Autodesk Inventor part; units mm, degrees
ref_plane "YZ Plane" through (0, 0, 0) normal (1, 0, 0) x (0, 1, 0)
ref_plane "XZ Plane" through (0, 0, 0) normal (0, 1, 0) x (-1, 0, 0)
ref_plane "XY Plane" through (0, 0, 0) normal (0, 0, 1) x (1, 0, 0)
sketch "Sketch1" plane through (0, 0, 0) normal (0, 0, 1) x (1, 0, 0)
  circle A0 centre (0, 0) radius 19.05
  circle A1 centre (0, 0) radius 9.906
  circle A2 centre (0, 0) radius 3
  dimension "d0" = 38.1
  dimension "d1" = 19.812
  dimension "d2" = 6
extrude "Extrusion1" add sketch "Sketch1" along normal blind 34.417 contours A0 | A1 | A2
extrude "Extrusion2" add sketch "Sketch1" against normal blind 5.207 contours A1
extrude "Extrusion3" add sketch "Sketch1" against normal blind 17.5768 contours A2
fillet "Fillet1" radius 1.5875 1 edges at (-19.05, 0, 34.417)
properties part number "OpticalRotaryEncoder"
Could you check a few things on this model? Use its own coordinates, in mm. A direction names the side the tool comes from. Give positions to 0.01 mm unless a question says otherwise; leave off trailing zeros. Order: outer loops, then holes, each group sorted by start corner. A loop starts at its lowest first (then second) coordinate and runs counter-clockwise, first axis right, second up. Notation, with made-up numbers: (79.25, 66.5) - (111.25, 66.5) arc R28 ccw to (111.25, 104.5) - close; hole circle Ø2 at (47, -6). An arc over 180 degrees is marked (long way). Return JSON: item names as keys, results as strings. Group by question number.
Q1. Which directions (+Z, -Z, +X, -X, +Y, -Y) give clear straight access to the entire face, cutting with the end or side of a thin tool? Please do faces 1 (the face through (-1.29, 9.82, -2.57)), 2 (the face through (0, 0, 34.417)).
Q2. Suppose I cut it at D-D, the plane z = -13. Please give me the cut outline in (x, y), and give its area (3 significant figures).
Q3. Suppose I cut it at C-C, the plane z = -2. Please give me the cut outline in (x, y).
Q4. Will these pins go through, and if not, where does the flat tip stop? pin 1 Ø3 at (x, z) = (-8, 16) entering from -Y; pin 2 Ø12 at (x, y) = (12.5, -14) entering from -Z; pin 3 Ø4 at (y, z) = (-0.5, -4.5) entering from -X.
Q5. Please list where these lines run through material, in increasing order: line 1 along Z through (x, y) = (-2.5, 12.5); line 2 along Z through (x, y) = (-0.5, 4); line 3 along Y through (x, z) = (0, -3). Write a range as [from, to].
Resolved:
{
 "1": {"face 1": "-Z", "face 2": "+Z, +X, -X, +Y, -Y"},
 "2": {"outline": "circle Ø6 at (0, 0)", "area": "28.3 mm2"},
 "3": {"outline": "circle Ø19.81 at (0, 0)"},
 "4": {"pin 1": "stops at y = -17.91", "pin 2": "stops at z = 0", "pin 3": "stops at x = -9.91"},
 "5": {"line 1": "z = [0, 34.42]", "line 2": "z = [-5.21, 34.42]", "line 3": "y = [-9.91, 9.91]"}
}
